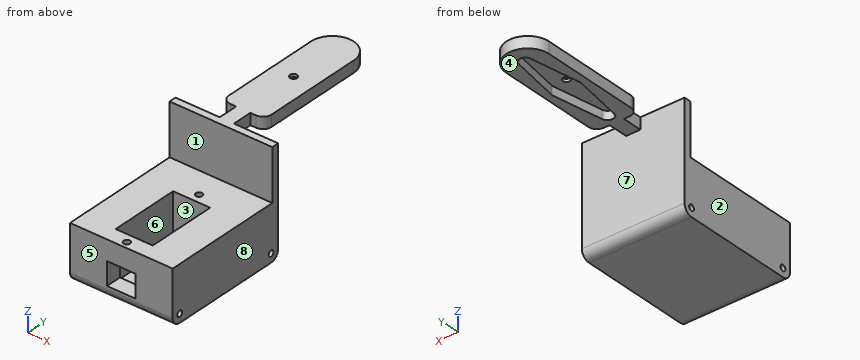
```python
from build123d import *

# Parameters (mm, degrees)
EXTRUDE_1_DEPTH     = 4
CUT_EXTRUDE_1_DEPTH = 3
SKETCH_5_R          = 1.25
CUT_EXTRUDE_2_DEPTH = 12.4
SKETCH_13_W         = 36
SKETCH_13_H         = 45
EXTRUDE_2_DEPTH     = 37
SKETCH_14_W         = 13
SKETCH_14_H         = 24.5
CUT_EXTRUDE_3_DEPTH = 35
SKETCH_15_R         = 1.15
CUT_EXTRUDE_4_DEPTH = 31
SKETCH_16_W         = 10
SKETCH_16_H         = 8
CUT_EXTRUDE_5_DEPTH = 8
SKETCH_17_W         = 36
SKETCH_17_H         = 42.5
CUT_EXTRUDE_6_DEPTH = 18
SKETCH_23_R         = 1.025
CUT_EXTRUDE_7_DEPTH = 5
SKETCH_24_R         = 1.025
CUT_EXTRUDE_8_DEPTH = 5
FILLET_1_R          = 3
FILLET_2_R          = 3
FILLET_3_R          = 3
FILLET_4_R          = 3


with BuildPart() as part:
    # 草圖1 → 填料-伸長1 (new body)
    with BuildSketch(Plane.XY):
        with BuildLine():
            Line((7.5, 17), (7.5, 55))
            ThreePointArc((7.5, 55), (0, 62.5), (-7.5, 55))
            Line((-7.5, 55), (-7.5, 17))
            Line((-7.5, 17), (-2.5, 17))
            Line((-2.5, 17), (-2.5, 15))
            Line((-2.5, 15), (-2.5, 10))
            Line((-2.5, 10), (2.5, 10))
            Line((2.5, 10), (2.5, 15))
            Line((2.5, 15), (2.5, 17))
            Line((2.5, 17), (7.5, 17))
        make_face()
    extrude(amount=EXTRUDE_1_DEPTH)

    # 草圖3 → 除料-伸長1 (cut)
    with BuildSketch(Plane.XY):
        with BuildLine():
            ThreePointArc((-2.132795501, 56), (0, 58.132795501), (2.132795501, 56))
            Line((2.132795501, 56), (5, 38.5))
            Line((5, 38.5), (2.114741289, 20.658021353))
            ThreePointArc((2.114741289, 20.658021353), (-0.171540182, 18.864665347), (-2.142213835, 21))
            Line((-2.142213835, 21), (-5, 38.5))
            Line((-5, 38.5), (-2.132795501, 56))
        make_face()
    extrude(amount=CUT_EXTRUDE_1_DEPTH, mode=Mode.SUBTRACT)

    # 草圖5 → 除料-伸長2 (cut)
    with BuildSketch(Plane.XY):
        with Locations((0, 38.5)):
            Circle(SKETCH_5_R)
    extrude(amount=CUT_EXTRUDE_2_DEPTH, mode=Mode.SUBTRACT)

    # 草圖13 → 填料-伸長2 (add)
    with BuildSketch(Plane.XY.offset(4)):
        with Locations((0, -12.5)):
            Rectangle(SKETCH_13_W, SKETCH_13_H)
    extrude(amount=-EXTRUDE_2_DEPTH)

    # 草圖14 → 除料-伸長3 (cut)
    with BuildSketch(Plane(origin=(0, 0, 4), x_dir=(-1, 0, 0), z_dir=(0, 0, -1))):
        with Locations((0, -17.25)):
            Rectangle(SKETCH_14_W, SKETCH_14_H)
    extrude(amount=CUT_EXTRUDE_3_DEPTH, mode=Mode.SUBTRACT)

    # 草圖15 → 除料-伸長4 (cut)
    with BuildSketch(Plane.XY.offset(4)):
        with Locations((0, -1.85)):
            Circle(SKETCH_15_R)
        with Locations((0, -32.65)):
            Circle(SKETCH_15_R)
    extrude(amount=-CUT_EXTRUDE_4_DEPTH, mode=Mode.SUBTRACT)

    # 草圖16 → 除料-伸長5 (cut)
    with BuildSketch(Plane(origin=(0, -35, 0), x_dir=(-1, 0, 0), z_dir=(0, -1, 0))):
        with Locations((0, 25)):
            Rectangle(SKETCH_16_W, SKETCH_16_H)
    extrude(amount=-CUT_EXTRUDE_5_DEPTH, mode=Mode.SUBTRACT)

    # 草圖17 → 除料-伸長6 (cut)
    with BuildSketch(Plane.XY.offset(4)):
        with Locations((0, -13.75)):
            Rectangle(SKETCH_17_W, SKETCH_17_H)
    extrude(amount=-CUT_EXTRUDE_6_DEPTH, mode=Mode.SUBTRACT)

    # 草圖23 → 除料-伸長7 (cut)
    with BuildSketch(Plane.ZY.offset(18)):
        with Locations((-30, 7)):
            Circle(SKETCH_23_R)
        with Locations((-30, -32)):
            Circle(SKETCH_23_R)
    extrude(amount=-CUT_EXTRUDE_7_DEPTH, mode=Mode.SUBTRACT)

    # 草圖24 → 除料-伸長8 (cut)
    with BuildSketch(Plane(origin=(18, 0, 0), x_dir=(0, 0, -1), z_dir=(1, 0, 0))):
        with Locations((30, 7)):
            Circle(SKETCH_24_R)
        with Locations((30, -32)):
            Circle(SKETCH_24_R)
    extrude(amount=-CUT_EXTRUDE_8_DEPTH, mode=Mode.SUBTRACT)

    # 圓角1
    fillet_1_edges = [part.edges().sort_by_distance(p)[0] for p in [
        (7.5, 17, 2),
    ]]
    fillet(fillet_1_edges, radius=FILLET_1_R)

    # 圓角2
    fillet_2_edges = [part.edges().sort_by_distance(p)[0] for p in [
        (-7.5, 17, 2),
    ]]
    fillet(fillet_2_edges, radius=FILLET_2_R)

    # 圓角3
    fillet_3_edges = [part.edges().sort_by_distance(p)[0] for p in [
        (0, 10, -33),
    ]]
    fillet(fillet_3_edges, radius=FILLET_3_R)

    # 圓角4
    fillet_4_edges = [part.edges().sort_by_distance(p)[0] for p in [
        (0, -35, -33),
    ]]
    fillet(fillet_4_edges, radius=FILLET_4_R)


solid = part.part
```
Can you work these out from the model? Positions are in its coordinate system, mm. Face numbers are marked on the shaded views. A direction names the side the tool comes from. Give positions to 0.01 mm unless a question says otherwise; leave off trailing zeros. Loops run counter-clockwise (first coordinate to the right, second up) from the corner with the lowest first, then second, coordinate; pieces in that order, holes last. Notation, with made-up numbers: M 51,-19.5 L 79,-19.5 A21 ccw 79,17.5 Z; hole C 19.5,-24.5 d8. An arc over 180 degrees is marked long. Answer in a Markdown table with one row per item.
1. Suppose I cut it at C-C on x = 14.5. Write out the boundary of the cut face in (y, z) (3 decimals), plus the area to 3 significant figures.
Taken from the geometry:
| item | result |
|---|---|
| outline | M -35,-30 A3 ccw -32,-33 L 7,-33 A3 ccw 10,-30 L 10,4 L 7.5,4 L 7.5,-14 L -35,-14 Z; hole C -32,-30 d2.05; hole C 7,-30 d2.05 |
| area | 890 mm² |
2. Suppose I cut it at A-A on x = 0. Count the separate pieces of the cut face and the enclosed holes in it, plus the area to 3 significant figures.
Taken from the geometry:
| item | result |
|---|---|
| separate pieces | 4 |
| enclosed holes | 0 |
| area | 479 mm² |
3. For pin 1 Ø6 at (x, y) = (-1, -31.5) entering from +Z; pin 2 Ø1.6 at (y, z) = (-32, -30) entering from +X; pin 3 Ø2 at (y, z) = (13.5, 1) entering from +X, each with a flat end and sliding along its axis, tell me the tip position at first contact or that it passes through.
Taken from the geometry:
| item | result |
|---|---|
| pin 1 | stops at z = -14 |
| pin 2 | stops at x = 13 |
| pin 3 | stops at x = 2.5 |
4. If I drill on line 1 along Y through (x, z) = (0, -18); line 2 along Y through (x, z) = (-15.85, -30) (3 decimals); line 3 along X through (y, z) = (-22, -29), over which ranges is the centre line in solid material (lowest first)?
Taken from the geometry:
| item | result |
|---|---|
| line 1 | y = -35 to -33.8, -31.5 to -29.5, -5 to -3, -0.7 to 10 |
| line 2 | y = -35 to -33.025, -30.975 to 5.975, 8.025 to 10 |
| line 3 | x = -18 to -6.5, 6.5 to 18 |
5. Suppose I cut it at D-D on z = -23. Write out the boundary of the cut face in (x, y).
Taken from the geometry:
| item | result |
|---|---|
| outline | M -18,-35 L -5,-35 L -5,-29.5 L -6.5,-29.5 L -6.5,-5 L 6.5,-5 L 6.5,-29.5 L 5,-29.5 L 5,-35 L 18,-35 L 18,10 L -18,10 Z; hole C 0,-1.85 d2.3 |
6. Suppose I cut it at B-B on z = -17. Write out the boundary of the cut face in (x, y).
Taken from the geometry:
| item | result |
|---|---|
| outline | M -18,-35 L 18,-35 L 18,10 L -18,10 Z; hole M -6.5,-29.5 L 6.5,-29.5 L 6.5,-5 L -6.5,-5 Z; hole C 0,-32.65 d2.3; hole C 0,-1.85 d2.3 |
7. Which directions (+Z, -Z, +X, -X, +Y, -Y) give clear straight access to the entire face, cutting with the end or side of a thin tool? Please do the marked faces 1, 2, 3, 4 and 5.
Taken from the geometry:
| item | result |
|---|---|
| face 1 | +Z, +X, -X, -Y |
| face 2 | +Z, -Z, -X, +Y, -Y |
| face 3 | +Z |
| face 4 | -Z, +X, -X, +Y |
| face 5 | +Z, -Z, +X, -X, -Y |
8. Thinking about a two-plate mould opening in X: for the marked faces 6, 7 and 8, which applies, released by +X, released by -X, zero draft, split by the parting line, or undercut?
Taken from the geometry:
| item | result |
|---|---|
| face 6 | undercut |
| face 7 | zero draft |
| face 8 | released by +X |
